Part model, mm, in its own coordinate system. Give positions to 0.01 mm unless a question says otherwise; leave off trailing zeros. Write each loop counter-clockwise with the first axis right and the second up, starting at its lowest first coordinate (ties: lowest second). Pieces come first, ordered by that corner, then holes.
```python
from build123d import *

# Parameters (mm, degrees)
SKETCH_2_W          = 120
SKETCH_2_H          = 110
SKETCH_2_R          = 1.6
EXTRUDE_1_DEPTH     = 3
SKETCH_4_W          = 90
SKETCH_4_H          = 198
EXTRUDE_2_DEPTH     = 3
SKETCH_7_W          = 5
SKETCH_7_H          = 3
SKETCH_7_W_2        = 3
SKETCH_7_H_2        = 5
CUT_EXTRUDE_1_DEPTH = 170.879368965
SKETCH_8_W          = 5
SKETCH_8_H          = 3
CUT_EXTRUDE_2_DEPTH = 170.879368965
SKETCH_9_W          = 5
SKETCH_9_H          = 40
CUT_EXTRUDE_3_DEPTH = 170.879368965
SKETCH_10_W         = 15
SKETCH_10_H         = 50
EXTRUDE_5_DEPTH     = 3
SKETCH_11_R         = 1.6
CUT_EXTRUDE_4_DEPTH = 170.879368965


with BuildPart() as part:
    # 草图2 → 凸台-拉伸1 (new body)
    with BuildSketch(Plane(origin=(0, 0, 0), x_dir=(1, 0, 0), z_dir=(0, 1, 0))):
        with Locations((55, 50)):
            Rectangle(SKETCH_2_W, SKETCH_2_H)
        with Locations(Location((0, 100, 0), (0, 0, 270))):
            Circle(SKETCH_2_R, mode=Mode.SUBTRACT)
        with Locations(Location((110, 100, 0), (0, 0, 270))):
            Circle(SKETCH_2_R, mode=Mode.SUBTRACT)
        with Locations(Location((0, 0, 0), (0, 0, 270))):
            Circle(SKETCH_2_R, mode=Mode.SUBTRACT)
        with Locations(Location((110, 0, 0), (0, 0, 270))):
            Circle(SKETCH_2_R, mode=Mode.SUBTRACT)
    extrude(amount=EXTRUDE_1_DEPTH)

    # 草图4 → 凸台-拉伸2 (add)
    with BuildSketch(Plane(origin=(0, 3, 0), x_dir=(1, 0, 0), z_dir=(0, 1, 0))):
        with Locations((55, 26)):
            Rectangle(SKETCH_4_W, SKETCH_4_H)
    extrude(amount=-EXTRUDE_2_DEPTH)

    # 草图7 → 切除-拉伸1 (cut, through all)
    with BuildSketch(Plane(origin=(0, 3, 0), x_dir=(1, 0, 0), z_dir=(0, 1, 0))):
        with Locations((24.5, 116.5)):
            Rectangle(SKETCH_7_W, SKETCH_7_H)
        with Locations((18.5, 107.5)):
            Rectangle(SKETCH_7_W_2, SKETCH_7_H_2)
    cut_extrude_1 = extrude(amount=-CUT_EXTRUDE_1_DEPTH, mode=Mode.SUBTRACT)

    # 镜向1: 切除-拉伸1 across plane
    add(cut_extrude_1.mirror(Plane.ZY.offset(-55)), mode=Mode.SUBTRACT)

    # 草图8 → 切除-拉伸2 (cut, through all)
    with BuildSketch(Plane(origin=(0, 3, 0), x_dir=(1, 0, 0), z_dir=(0, 1, 0))):
        with Locations((55, -54.5)):
            Rectangle(SKETCH_8_W, SKETCH_8_H)
    extrude(amount=-CUT_EXTRUDE_2_DEPTH, mode=Mode.SUBTRACT)

    # 草图9 → 切除-拉伸3 (cut, through all)
    with BuildSketch(Plane(origin=(0, 3, 0), x_dir=(1, 0, 0), z_dir=(0, 1, 0))):
        with Locations((17.5, 50)):
            Rectangle(SKETCH_9_W, SKETCH_9_H)
        with Locations((92.5, 50)):
            Rectangle(SKETCH_9_W, SKETCH_9_H)
    extrude(amount=-CUT_EXTRUDE_3_DEPTH, mode=Mode.SUBTRACT)

    # 草图10 → 凸台-拉伸5 (add)
    with BuildSketch(Plane(origin=(0, 3, 0), x_dir=(1, 0, 0), z_dir=(0, 1, 0))):
        with Locations((2.5, -30)):
            Rectangle(SKETCH_10_W, SKETCH_10_H)
        with Locations((107.5, -30)):
            Rectangle(SKETCH_10_W, SKETCH_10_H)
    extrude(amount=-EXTRUDE_5_DEPTH)

    # 草图11 → 切除-拉伸4 (cut, through all)
    with BuildSketch(Plane(origin=(0, 3, 0), x_dir=(1, 0, 0), z_dir=(0, 1, 0))):
        with Locations(Location((0, -50, 0), (0, 0, 270))):
            Circle(SKETCH_11_R)
        with Locations(Location((0, 65, 0), (0, 0, 270))):
            Circle(SKETCH_11_R)
        with Locations(Location((110, -50, 0), (0, 0, 270))):
            Circle(SKETCH_11_R)
        with Locations(Location((110, 65, 0), (0, 0, 270))):
            Circle(SKETCH_11_R)
    extrude(amount=-CUT_EXTRUDE_4_DEPTH, mode=Mode.SUBTRACT)


solid = part.part
```
1) Saw through at A-A, the plane z = -58. Write the cut outline in (x, y), then the cut area to 3 significant figures.
Answers follow:
outline: (-5, 0) - (15, 0) - (15, 3) - (-5, 3) - close; (20, 0) - (90, 0) - (90, 3) - (20, 3) - close; (95, 0) - (115, 0) - (115, 3) - (95, 3) - close
area: 330 mm2
2) Wall check: L1, parallel to X at y = 0.9, z = -59; L2, parallel to X at y = 1.15, z = 0; L3, parallel to Z at x = 110, y = 0.8. Give the ranges that are in metal, low to high.
Answers follow:
L1: x = -5 to 15, 20 to 90, 95 to 115
L2: x = -5 to -1.6, 1.6 to 108.4, 111.6 to 115
L3: z = -105 to -101.6, -98.4 to -66.6, -63.4 to -1.6, 1.6 to 48.4, 51.6 to 55
3) Saw through at B-B, the plane y = 2.15. Count the separate pieces of the cut face and the enclosed holes in it, then the cut area to 3 significant figures.
Answers follow:
separate pieces: 1
enclosed holes: 15
area: 22,100 mm2
4) Pin check, flat tips, straight feed: pin 1 Ø0.9 at (y, z) = (1.5, 64) entering from +X; pin 2 Ø1.5 at (x, y) = (105.5, 1) entering from +Z. Stop position of each tip, or through.
Answers follow:
pin 1: stops at x = 100
pin 2: stops at z = 55
